```python
from build123d import *

# Parameters (mm, degrees)
SKETCH1_R                    = 175
BOSS_EXTRUDE3_DEPTH          = 30
CUT_EXTRUDE1_DEPTH           = 50
SHELL2_T                     = -3
SKETCH4_R                    = 10
CUT_EXTRUDE2_DEPTH           = 50
FILLET1_R                    = 10
SKETCH6_R                    = 50
CUT_EXTRUDE4_DEPTH           = 10
SKETCH9_W                    = 50
SKETCH9_H                    = 20
BOSS_EXTRUDE4_DEPTH          = 20
F_5_0_5_DIAMETER_HOLE2_D     = 5
F_5_0_5_DIAMETER_HOLE2_DEPTH = 11
F_5_0_5_DIAMETER_HOLE2_TIP   = 1.502151548


with BuildPart() as part:
    # Sketch1 → Boss-Extrude3 (new body)
    with BuildSketch(Plane.XY):
        Circle(SKETCH1_R)
    extrude(amount=BOSS_EXTRUDE3_DEPTH)

    # Sketch3 → Cut-Extrude1 (cut)
    with BuildSketch(Plane.XY.offset(30)):
        with BuildLine():
            Line((-175, 0), (175, 0))
            ThreePointArc((175, 0), (0, -175), (-175, 0))
        make_face()
    extrude(amount=-CUT_EXTRUDE1_DEPTH, mode=Mode.SUBTRACT)

    # Shell2
    shell2_openings = [part.faces().sort_by_distance(p)[0] for p in [
        (0, 0, 15),
    ]]
    offset(amount=SHELL2_T, openings=shell2_openings)

    # Sketch4 → Cut-Extrude2 (cut)
    with BuildSketch(Plane.XY.offset(30)):
        Circle(SKETCH4_R)
    extrude(amount=-CUT_EXTRUDE2_DEPTH, mode=Mode.SUBTRACT)

    # Fillet1
    fillet1_edges = [part.edges().sort_by_distance(p)[0] for p in [
        (0, 175, 0),
        (0, 175, 30),
    ]]
    fillet(fillet1_edges, radius=FILLET1_R)

    # Sketch6 → Cut-Extrude4 (cut)
    with BuildSketch(Plane(origin=(0, 0, 0), x_dir=(-1, 0, 0), z_dir=(0, 0, -1))):
        Circle(SKETCH6_R)
    extrude(amount=-CUT_EXTRUDE4_DEPTH, mode=Mode.SUBTRACT)

    # Sketch9 → Boss-Extrude4 (add)
    with BuildSketch(Plane.XY.offset(30)):
        with Locations((-90, 38)):
            Rectangle(SKETCH9_W, SKETCH9_H)
    boss_extrude4 = extrude(amount=BOSS_EXTRUDE4_DEPTH)

    # Mirror2: Boss-Extrude4 across plane
    add(boss_extrude4.mirror(Plane(origin=(0, 0, 0), x_dir=(0, 0, 1), z_dir=(1, 0, 0))))

    # Ø5.0 (5) Diameter Hole2
    with Locations(Plane.XY.offset(50)):
        with Locations((-100, 38), (-80, 38), (80, 38), (100, 38)):
            Hole(F_5_0_5_DIAMETER_HOLE2_D / 2, depth=F_5_0_5_DIAMETER_HOLE2_DEPTH)
            with Locations((0, 0, -(F_5_0_5_DIAMETER_HOLE2_DEPTH + F_5_0_5_DIAMETER_HOLE2_TIP / 2))):  # 118° drill point
                Cone(0, F_5_0_5_DIAMETER_HOLE2_D / 2, F_5_0_5_DIAMETER_HOLE2_TIP, mode=Mode.SUBTRACT)


solid = part.part
```
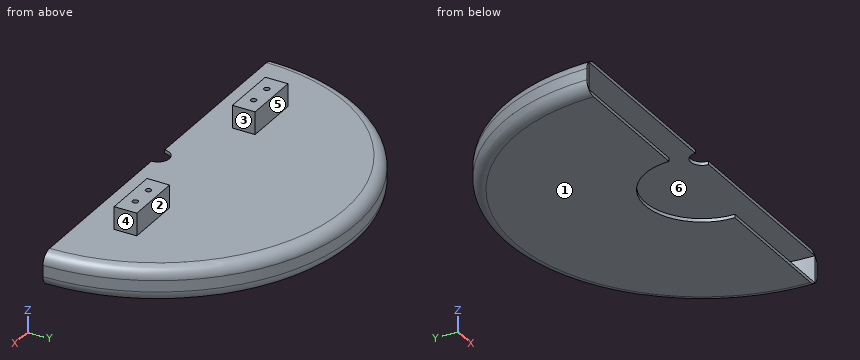
The listing builds one solid part. Answer for the finished solid, in the listing's coordinates (mm). Face numbers are marked on the shaded views. A direction names the side the tool comes from. Coordinates: 2 decimals unless noted, no trailing zeros. Loops run counter-clockwise (first coordinate to the right, second up) from the corner with the lowest first, then second, coordinate; pieces in that order, holes last. Notation, with made-up numbers: (0, -15) - (30, -15) arc R18 ccw to (30, -3) - close; hole circle Ø11 at (16, 1). An arc over 180 degrees is marked (long way). Write item = value, one per line.
1) Find the intervals of material crossed by line 1 along X through (y, z) = (38, 45); line 2 along Y through (x, z) = (80, 44.75); line 3 along Z through (x, y) = (52, 72), in increasing order.
Responses:
line_1 = -115 to -102.5, -97.5 to -82.5, -77.5 to -65, 65 to 77.5, 82.5 to 97.5, 102.5 to 115
line_2 = 28 to 35.5, 40.5 to 48
line_3 = 0 to 3, 27 to 30
2) Each of these flat-tipped pins is pushed along its axis until it touches: P1, Ø12, axis at y = 102, z = 7.5, coming from the -X side; P2, Ø10, axis at x = -79, z = 41, coming from the -Y side; P3, Ø6, axis at y = 130, z = 28, coming from the -X side. Where does it stop, or does it pass through?
Responses:
P1 = -146.14
P2 = 28
P3 = -116.65
3) Section A-A (z = 44.5) is taken. Determine the outline of the cut face in (x, y), plus the area to 3 significant figures.
Responses:
outline = (-115, 28) - (-65, 28) - (-65, 48) - (-115, 48) - close; (65, 28) - (115, 28) - (115, 48) - (65, 48) - close; hole circle Ø5 at (-100, 38); hole circle Ø5 at (-80, 38); hole circle Ø5 at (80, 38); hole circle Ø5 at (100, 38)
area = 1,920 mm^2
4) Which of the six approach directions +Z, -Z, +X, -X, +Y, -Y give full straight-line access (tool end or side, diameter ignored) to the marked faces 1, 2 and 3?
Responses:
face_1 = -Z, +X, -X, +Y, -Y
face_2 = +Z, +X, -X, +Y
face_3 = +Z, +Y, -Y
5) Determine the mould class of the marked faces 4, 5 and 6 for opening direction X: pulls with the +X half, pulls with the -X half, needs draft (parallel to the pull), parting line crosses it, or undercut.
Responses:
face_4 = pulls with the +X half
face_5 = needs draft
face_6 = undercut
6) Section B-B (x = 0) is taken. Determine the outline of the cut face in (y, z), plus the area to 3 significant figures.
Responses:
outline = (10, 27) - (172, 27) - (172, 3) - (50, 3) - (50, 0) - (165, 0) arc R10 ccw to (175, 10) - (175, 20) arc R10 ccw to (165, 30) - (10, 30) - close
area = 899 mm^2
